The model under review builds one solid part; all positions refer to its coordinate system, in mm. Face numbers are marked on the shaded views. A direction names the side the tool comes from. Give positions to 0.01 mm unless a question says otherwise; leave off trailing zeros. Order: outer loops, then holes, each group sorted by start corner. A loop starts at its lowest first (then second) coordinate and runs counter-clockwise, first axis right, second up.
Autodesk Inventor part; units mm, degrees
ref_plane "YZ Plane" through (0, 0, 0) normal (1, 0, 0) x (0, 1, 0)
ref_plane "XZ Plane" through (0, 0, 0) normal (0, 1, 0) x (-1, 0, 0)
ref_plane "XY Plane" through (0, 0, 0) normal (0, 0, 1) x (1, 0, 0)
sketch "Sketch7" plane through (0, 0, 0) normal (0, 1, 0) x (-1, 0, 0)
  line L0 (0, 0) -> (-22.225, 0)
  line L1 (0, 0) -> (-15.7154, -15.7154) construction
  line L2 (0, 0) -> (-22.225, 0) construction
  line L3 (-22.225, 0) -> (-19.8975, -9.9016)
  line L4 (-19.8975, -9.9016) -> (-15.7154, -15.7154)
  line L5 (-15.7154, -15.7154) -> (0, 0)
  dimension "d25" = 22.225
  dimension "d26" = 45
extrude "Extrusion6" add sketch "Sketch7" along normal blind 19.05
chamfer "Chamfer2" distance 19.05 angle 45 2 edges at (17.8065, 19.05, -12.8085) (21.0612, 19.05, -4.9508)
pattern_circular "Circular Pattern3" count 8 over 360 about axis through (0, 0, 0) along (0, 1, 0) of "Extrusion6", "Chamfer2"
sketch "Sketch8" plane through (-15.7154, 0, -15.7154) normal (-0.6011477, 0.7071068, -0.372319) x (0.5066767, 0.6975367, 0.5066767)
  line L0 (0, 0) -> (1.6678, -10.0338)
  line L1 (1.6678, -10.0338) -> (27.6226, -1.8784)
  line L2 (27.6226, -1.8784) -> (1.6678, -10.0338)
  line L3 (27.6226, -1.8784) -> (27.3104, 0)
  line L4 (27.3104, 0) -> (0, 0)
  line L5 (0, 0) -> (27.3104, 0)
  point P0 (15.9253, -2.5084)
extrude "Extrusion7" add sketch "Sketch8" along normal blind 6.35 draft -23.6
sketch "Sketch9" plane through (0, 0, 0) normal (0, -1, 0) x (1, 0, 0)
  circle A0 centre (0, 0) radius 4.7625
  dimension "d37" = 9.525
extrude "Extrusion8" add sketch "Sketch9" along normal blind 12.7
pattern_circular "Circular Pattern4" count 8 over 360 about axis through (0, 0, 0) along (0, -1, 0) of "Extrusion7"
properties part number "Beveled_Gear"
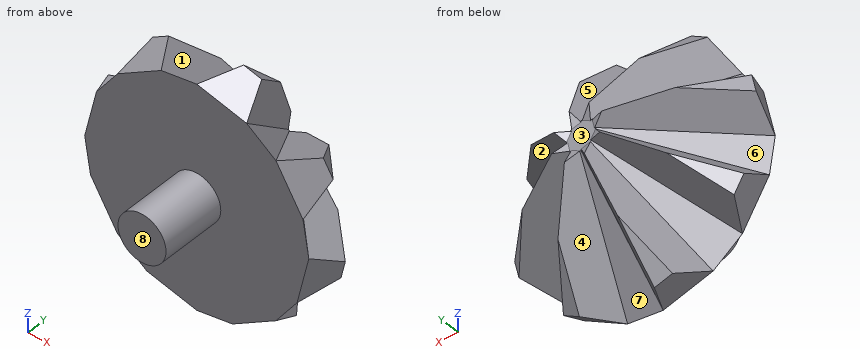
1. Take a section at A-A (z = -12.5). Write out the cut boundary in (x, y), and give its area (3 significant figures).
2. Take a section at C-C (x = 17.5). Write out the cut boundary in (y, z).
3. Draft analysis for pull direction X (two halves, no side actions). For the marked faces 5, 6, 7 and 8, state which applies: pulls with the +X half, pulls with the -X half, needs draft (parallel to the pull), parting line crosses it, or undercut.
4. To check wall thickness, follow line 1 (Y direction, x = 17, z = -7); line 2 (X direction, y = 4.5, z = 20); line 3 (X direction, y = 13.5, z = -13). State the ranges of each line that lie inside material, in increasing order.
5. Insertion check: pin 1 (4 mm diameter, centred on x = -17, y = 15, fed in from -Z); pin 2 (1.5 mm diameter, centred on y = -2, z = 0.5, fed in from +X); pin 3 (3 mm diameter, centred on x = -9, z = 18, fed in from -Y). Each pin has a flat end and moves straight along its axis. Give the tip position at first contact, or say it passes through.
6. Take a section at B-B (y = -3). Write out the cut boundary in (x, z) (1 decimal), and give its area (3 significant figures).
7. For the marked faces 1, 2, 3 and 4, list the 3-axis set-ups (+Z, -Z, +X, -X, +Y, -Y) from which the entire face can be reached by the end or side of a thin tool; tool diameter is ignored.
Answer:
1. outline: (-20.68, 6.45) - (-17.71, 0) - (18.03, 0) - (12.5, 4.49) - (12.5, 4.43) - (7.5, 15.5) - (3.86, 8.98) - (0, 9.6) - (0, 9.47) - (-3.18, 16.31) - (-6.53, 7.97) - (-12.5, 4.49) - (-12.5, 4.43) - (-17.82, 8.88) - close
1. area: 309 mm2
2. outline: (0, -13.23) - (2.58, -8.81) - (12.47, -4.83) - (12.72, -3.77) - (4.6, 0) - (4.66, 0) - (3.74, 5.73) - (10.68, 9.6) - (9.33, 12.18) - (2.97, 15.05) - (0, 12.83) - close
3. face 5: undercut
3. face 6: pulls with the -X half
3. face 7: undercut
3. face 8: needs draft
4. line 1: y = 0 to 7.05
4. line 2: x = -12.15 to -8.55, 1.08 to 8.09
4. line 3: x = -4.32 to -2.1, 6.86 to 8.59
5. pin 1: stops at z = 3.3
5. pin 2: stops at x = 4.76
5. pin 3: stops at y = 0
6. outline: circle Ø9.5 at (0, 0)
6. area: 71.3 mm2
7. face 1: +Z, +Y
7. face 2: +X, +Y
7. face 3: +Y
7. face 4: -Z, +Y
